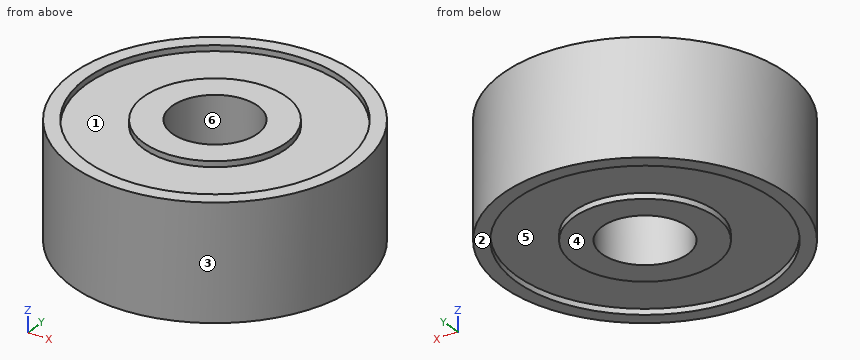
Solid Edge part; units mm, degrees
sketch "Sketch1" plane through (0, 0, 0) normal (0, 0, 1) x (1, 0, 0)
  circle A0 centre (0, 0) radius 1.5
  circle A1 centre (0, 0) radius 5
extrude "Protrusion1" add sketch "Sketch1" along normal blind 4
sketch "Sketch2" plane through (0, 0, 0) normal (0, -1, 0) x (1, 0, 0)
  line L0 (0, 4) -> (2.5, 4)
  line L1 (2.5, 4) -> (2.5, 3.8)
  line L2 (2.5, 3.8) -> (4.5, 3.8)
  line L3 (4.5, 3.8) -> (4.5, 4)
  line L4 (4.5, 4) -> (5.6166, 4)
revolve "RevolvedCutout1" cut sketch "Sketch2" angle 360 about axis through (0, 0, 54) along (0, 0, -1) material side at (1.25, 0, 4.05)
mirror "Mirror1" about plane through (0, 0, 2) normal (0, 0, 1) of "RevolvedCutout1"
properties material "Stainless steel"
Design review of the part built by this model. Coordinates are the model's own, in mm. Face numbers are marked on the shaded views. A direction names the side the tool comes from. Coordinates: 2 decimals unless noted, no trailing zeros. Order: outer loops, then holes, each group sorted by start corner. A loop starts at its lowest first (then second) coordinate and runs counter-clockwise, first axis right, second up. Notation, with made-up numbers: (57.25, 8) -> (112.25, 8) arc R34 ccw to (112.25, 42) -> close; hole circle Ø10 at (-7, 3). An arc over 180 degrees is marked (long way). One line per item, written item: value. Start each with the question number.
Q1. Mouldability with a two-part tool opening along Y and no side actions: class the marked faces 3, 4, 5 and 6 as pulls with the +Y half, pulls with the -Y half, needs draft (parallel to the pull), parting line crosses it, or undercut.
Q2. Take a section at C-C, the plane z = 2.05. State the section outline as (x, y) points, then the cut area to 3 significant figures.
Q3. For probe 1 along Y at (x, z) = (0, 0.05); probe 2 along Y at (x, z) = (0, 3.2); probe 3 along Y at (x, z) = (-1, 3.15), list the stretches that pass through material, from the lowest coordinate up.
Q4. Take a section at A-A, the plane x = 0. State the section outline as (y, z) points, then the cut area to 3 significant figures.
Q5. Insertion check: pin 1 Ø2 at (x, y) = (-1, -1) entering from +Z; pin 2 Ø1 at (x, z) = (-2, 2) entering from -Y; pin 3 Ø1.5 at (x, z) = (1, 1) entering from -Y. Each pin has a flat end and moves straight along its axis. Give the tip position at first contact, or say it passes through.
Q6. Tool access review of the marked faces 1 and 2: name each direction out of +Z, -Z, +X, -X, +Y, -Y from which nothing blocks a thin tool from reaching the whole face with its end or side.
Q7. Take a section at D-D, the plane y = -2.25. State the section outline as (x, z) points.
Values follow:
1. face 3: parting line crosses it
1. face 4: needs draft
1. face 5: undercut
1. face 6: undercut
2. outline: circle Ø10 at (0, 0); hole circle Ø3 at (0, 0)
2. area: 71.5 mm2
3. probe 1: y = -5 to -4.5, -2.5 to -1.5, 1.5 to 2.5, 4.5 to 5
3. probe 2: y = -5 to -1.5, 1.5 to 5
3. probe 3: y = -4.9 to -1.12, 1.12 to 4.9
4. outline: (-5, 0) -> (-4.5, 0) -> (-4.5, 0.2) -> (-2.5, 0.2) -> (-2.5, 0) -> (-1.5, 0) -> (-1.5, 4) -> (-2.5, 4) -> (-2.5, 3.8) -> (-4.5, 3.8) -> (-4.5, 4) -> (-5, 4) -> close; (1.5, 0) -> (2.5, 0) -> (2.5, 0.2) -> (4.5, 0.2) -> (4.5, 0) -> (5, 0) -> (5, 4) -> (4.5, 4) -> (4.5, 3.8) -> (2.5, 3.8) -> (2.5, 4) -> (1.5, 4) -> close
4. area: 26.4 mm2
5. pin 1: stops at z = 4
5. pin 2: stops at y = -4.77
5. pin 3: stops at y = -4.99
6. face 1: +Z
6. face 2: -Z, +X, -X, +Y, -Y
7. outline: (-4.47, 0) -> (-3.9, 0) -> (-3.9, 0.2) -> (-1.09, 0.2) -> (-1.09, 0) -> (1.09, 0) -> (1.09, 0.2) -> (3.9, 0.2) -> (3.9, 0) -> (4.47, 0) -> (4.47, 4) -> (3.9, 4) -> (3.9, 3.8) -> (1.09, 3.8) -> (1.09, 4) -> (-1.09, 4) -> (-1.09, 3.8) -> (-3.9, 3.8) -> (-3.9, 4) -> (-4.47, 4) -> close
